Part print with two shaded views. Sizes in mm from the minimum x, y, z corner. Round coordinates to 2 decimals unless told otherwise and drop trailing zeros. Loops run counter-clockwise (first coordinate to the right, second up) from the corner with the lowest first, then second, coordinate; pieces in that order, holes last.
(1) Probe probe 1 along Z at (x, y) = (10, 1); probe 2 along Z at (x, y) = (12, 3.25). List the from-to ranges inside material, lowest first.
(2) Cut at D-D on y = 2.3. List the corners of the cut face in (x, z).
(3) Cut at B-B on z = 10. List the corners of the cut face in (x, y).
(4) Cut at C-C on x = 30. List the corners of the cut face in (y, z), then the cut area to 3 significant figures.
(5) Flat gauge pins, fed straight in: pin 1 (7 mm diameter, centred on x = 50, z = 10, fed in from -Y); pin 2 (2 mm diameter, centred on x = 39.5, y = 2, fed in from +Z). Where does each tip first touch, or does it go through?
(6) Cut at A-A on z = 50. List the corners of the cut face in (x, y), then the cut area to 3 significant figures.
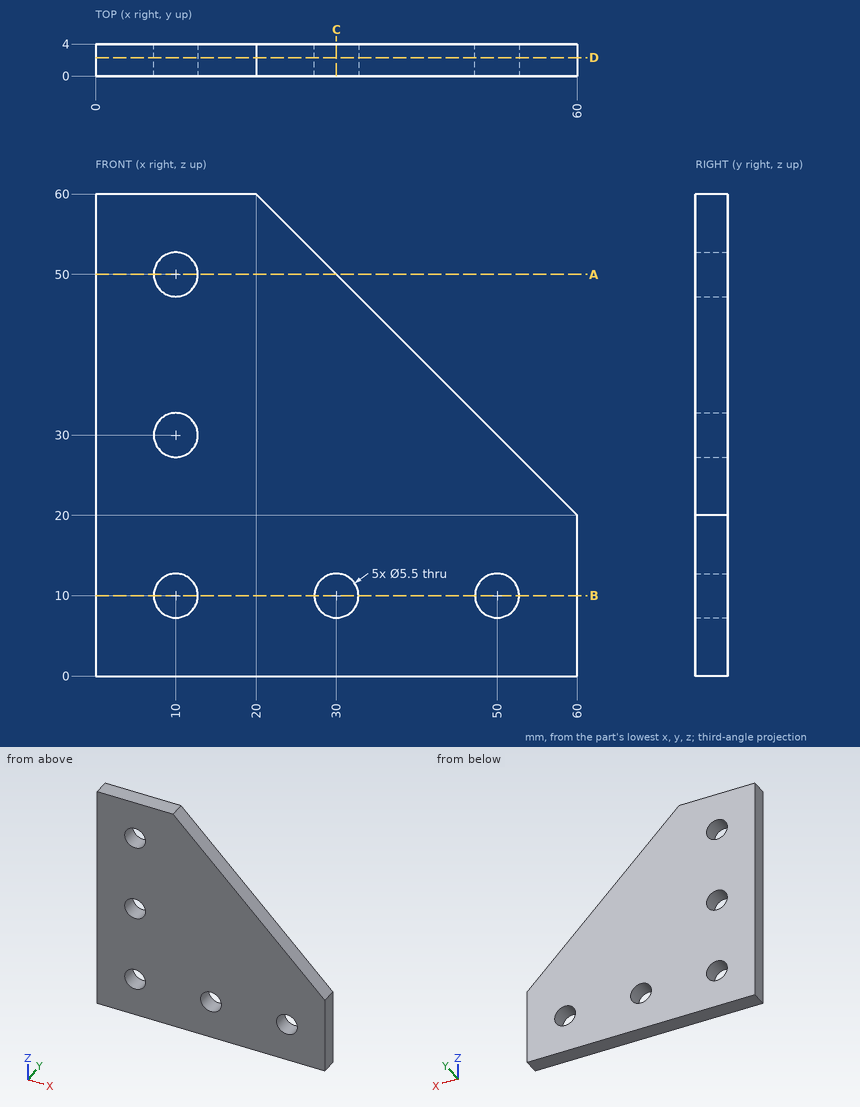
Final values:
1. probe 1: z = 0 to 7.25, 12.75 to 27.25, 32.75 to 47.25, 52.75 to 60
1. probe 2: z = 0 to 8.11, 11.89 to 28.11, 31.89 to 48.11, 51.89 to 60
2. outline: (0, 0) - (60, 0) - (60, 20) - (20, 60) - (0, 60) - close; hole circle Ø5.5 at (10, 10); hole circle Ø5.5 at (10, 30); hole circle Ø5.5 at (10, 50); hole circle Ø5.5 at (30, 10); hole circle Ø5.5 at (50, 10)
3. outline: (0, 0) - (7.25, 0) - (7.25, 4) - (0, 4) - close; (12.75, 0) - (27.25, 0) - (27.25, 4) - (12.75, 4) - close; (32.75, 0) - (47.25, 0) - (47.25, 4) - (32.75, 4) - close; (52.75, 0) - (60, 0) - (60, 4) - (52.75, 4) - close
4. outline: (0, 0) - (4, 0) - (4, 7.25) - (0, 7.25) - close; (0, 12.75) - (4, 12.75) - (4, 50) - (0, 50) - close
4. area: 178 mm2
5. pin 1: stops at y = 0
5. pin 2: stops at z = 41.5
6. outline: (0, 0) - (7.25, 0) - (7.25, 4) - (0, 4) - close; (12.75, 0) - (30, 0) - (30, 4) - (12.75, 4) - close
6. area: 98.0 mm2
